Geometry: see drawing. Coordinates: mm, zero at the bounding-box minimum. Give positions to 0.01 mm unless a question says otherwise; leave off trailing zeros. Order: outer loops, then holes, each group sorted by start corner. A loop starts at its lowest first (then second) coordinate and runs counter-clockwise, first axis right, second up. Notation, with made-up numbers: (81.5, 5) - (112.5, 5) arc R10 cw to (112.5, 22) - close; hole circle Ø1 at (-20.75, -13.5). An arc over 180 degrees is marked (long way). Put each result on its own line as item: value. Start each with the question number.
1. Section B-B on y = 14. Return the cut outline in (x, z) (3 decimals).
2. First-contact query: P1, Ø0.8, axis at y = 36, z = 1, coming from the +X side; P2, Ø2, axis at x = 42.5, y = 51, coming from the -Z side. Flat tips, straight axial feed; report the tip coordinate or a pass-through.
3. Ray query, line 1 along Y through (x, z) = (36, 0.55) (3 decimals); line 2 along X through (y, z) = (7.5, 0.8); line 3 along Y through (x, z) = (3.5, 0.4). Return the intervals inside material, ascending. Write a range as from..to.
4. Section D-D on x = 73. Return the cut outline in (y, z).
5. Section A-A on z = 0.65. Return the cut outline in (x, y) (3 decimals), plus the area to 3 significant figures.
6. Section C-C on x = 36. Return the cut outline in (y, z) (3 decimals), plus the area to 3 significant figures.
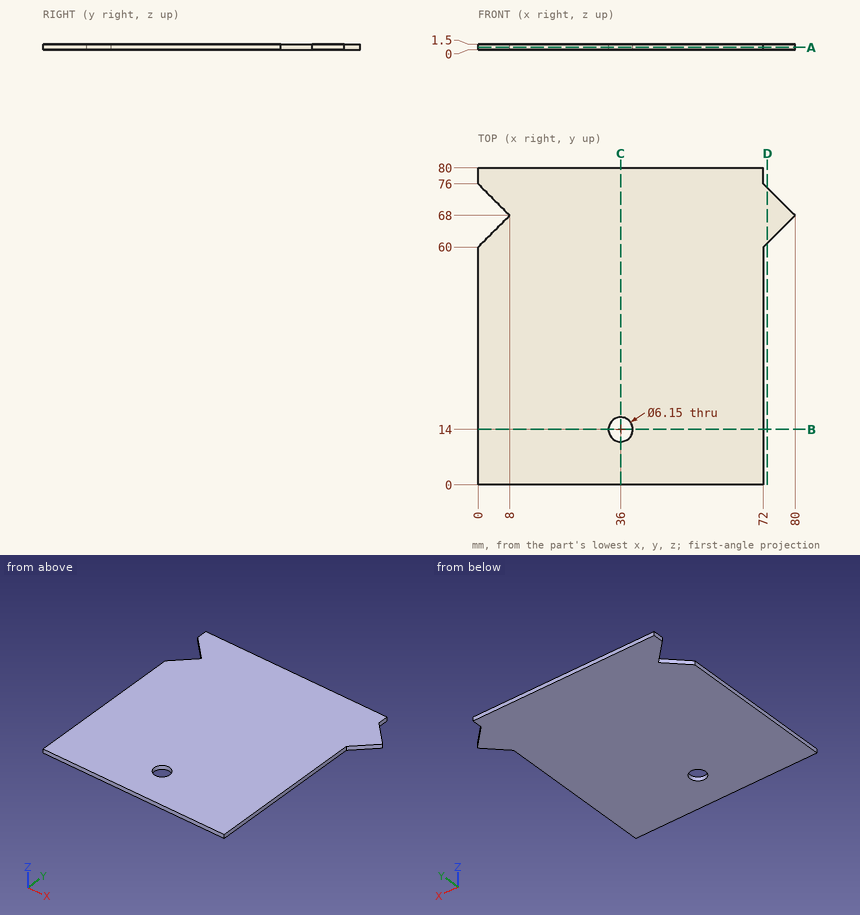
Resolved:
1. outline: (0, 0) - (32.925, 0) - (32.925, 1.5) - (0, 1.5) - close; (39.075, 0) - (72, 0) - (72, 1.5) - (39.075, 1.5) - close
2. P1: x = 72
2. P2: z = 0
3. line 1: 0..10.925, 17.075..80
3. line 2: 0..72
3. line 3: 0..63.5, 72.5..80
4. outline: (61, 0) - (75, 0) - (75, 1.5) - (61, 1.5) - close
5. outline: (0, 0) - (72, 0) - (72, 60) - (80, 68) - (72, 76) - (72, 80) - (0, 80) - (0, 76) - (8, 68) - (0, 60) - close; hole circle Ø6.15 at (36, 14)
5. area: 5,730 mm^2
6. outline: (0, 0) - (10.925, 0) - (10.925, 1.5) - (0, 1.5) - close; (17.075, 0) - (80, 0) - (80, 1.5) - (17.075, 1.5) - close
6. area: 111 mm^2
